Autodesk Inventor part; units mm, degrees
ref_plane "YZ Plane" through (0, 0, 0) normal (1, 0, 0) x (0, 1, 0)
ref_plane "XZ Plane" through (0, 0, 0) normal (0, 1, 0) x (-1, 0, 0)
ref_plane "XY Plane" through (0, 0, 0) normal (0, 0, 1) x (1, 0, 0)
sketch "Sketch1" plane through (0, 0, 0) normal (1, 0, 0) x (0, 1, 0)
  circle A0 centre (0, 0) radius 12.7
  dimension "d0" = 25.4
extrude "Extrusion1" add sketch "Sketch1" along normal blind 19.05
chamfer "Chamfer1" distance 1.143 angle 45 1 edges at (19.05, -12.7, 0)
sketch "Sketch2" plane through (0, 0, 0) normal (-1, 0, 0) x (0, 0, 1)
  circle A0 centre (0, 0) radius 12.7
ref_plane "Work Plane1" through (-29.21, 0, 0) normal (-1, 0, 0) x (0, 0, 1)
sketch "Sketch3" plane through (-29.21, 0, 0) normal (-1, 0, 0) x (0, 0, 1)
  circle A0 centre (0, 0) radius 6.096
  dimension "d7" = 12.192
loft "Loft1" add profiles "Sketch3" section 1 edges at (0, -12.7, 0)
sketch "Sketch4" plane through (-29.21, 0, 0) normal (-1, 0, 0) x (0, 0, 1)
  circle A0 centre (0, 0) radius 4.7625
  dimension "d12" = 9.525
extrude "Extrusion2" add sketch "Sketch4" along normal blind 15.24
properties part number "Kevin_CAD_test_2"
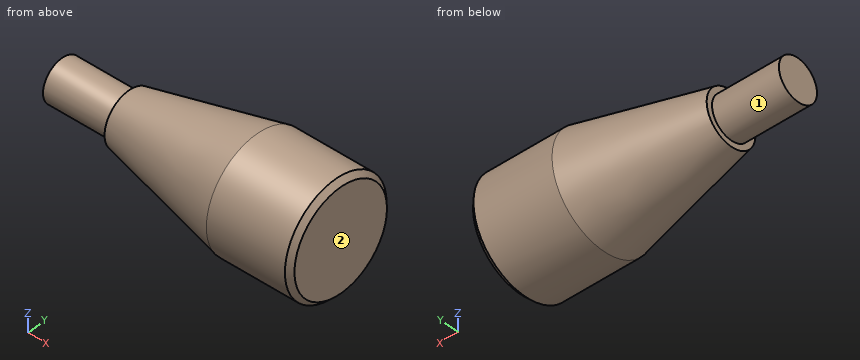
Input: part model. Units: mm. Frame: model coordinates. Face numbers are marked on the shaded views. A direction names the side the tool comes from. Round coordinates to 2 decimals unless told otherwise and drop trailing zeros. Write each loop counter-clockwise with the first axis right and the second up, starting at its lowest first coordinate (ties: lowest second). Pieces come first, ordered by that corner, then holes.
1) Reachability of the marked faces 1 and 2 from +Z, -Z, +X, -X, +Y, -Y: full face, straight path, thin tool, end or side. Return the list, or none.
2) Cut plane A-A (y = 0). Return the cut outline in (x, z), then the cut area to 3 significant figures.
3) Cut plane B-B (x = 2). Return the cut outline in (y, z).
4) Ray query, L1, parallel to Z at x = -17.5, y = -7.5; L2, parallel to Z at x = -21, y = -2; L3, parallel to X at y = 4, z = 4.25. Return the intervals inside material, ascending.
5) Contact query for flat-ended pins moving along their axis: P1, Ø8, axis at x = -13.5, y = 2.5, coming from the -Z side; P2, Ø1.5, axis at x = -35.5, z = -5, coming from the +Y side; P3, Ø10, axis at x = -21.5, z = -10, coming from the +Y side. Output: stop coordinate, or through.
6) Cut plane C-C (x = -31). Return the cut outline in (y, z) (1 decimal), then the cut area to 3 significant figures.
Geometry says:
1. face 1: -X
1. face 2: +Z, -Z, +X, +Y, -Y
2. outline: (-44.45, -4.76) - (-29.21, -4.76) - (-29.21, -6.1) - (0, -12.7) - (17.91, -12.7) - (19.05, -11.56) - (19.05, 11.56) - (17.91, 12.7) - (0, 12.7) - (-29.21, 6.1) - (-29.21, 4.76) - (-44.45, 4.76) - close
2. area: 1,180 mm2
3. outline: circle Ø25.4 at (0, 0)
4. L1: z = -4.49 to 4.49
4. L2: z = -7.7 to 7.7
4. L3: x = -29.21 to 19.05
5. P1: stops at z = -10.44
5. P2: stops at y = 2.15
5. P3: stops at y = 6.29
6. outline: circle Ø9.5 at (0, 0)
6. area: 71.3 mm2
